Can you work these out from the model? Positions are in its coordinate system, mm. Face numbers are marked on the shaded views. A direction names the side the tool comes from. Give positions to 0.01 mm unless a question says otherwise; leave off trailing zeros. Write each loop counter-clockwise with the first axis right and the second up, starting at its lowest first coordinate (ties: lowest second). Pieces come first, ordered by that corner, then holes.
```python
from build123d import *

# Parameters (mm, degrees)
SKETCH1_W           = 54
SKETCH1_H           = 26.5
BOSS_EXTRUDE1_DEPTH = 9
SKETCH2_W           = 6
SKETCH2_H           = 15
BOSS_EXTRUDE2_DEPTH = 19
SKETCH4_R           = 2.06
CUT_EXTRUDE1_DEPTH  = 19
SKETCH5_R           = 2.06
BOSS_EXTRUDE3_DEPTH = 15
SKETCH8_W           = 54
SKETCH8_H           = 10
BOSS_EXTRUDE5_DEPTH = 9
SKETCH9_R           = 2.25
CUT_EXTRUDE3_DEPTH  = 15
FILLET1_R           = 2
FILLET2_R           = 1


with BuildPart() as part:
    # Sketch1 → Boss-Extrude1 (new body)
    with BuildSketch(Plane.XY):
        Rectangle(SKETCH1_W, SKETCH1_H)
    boss_extrude1 = extrude(amount=BOSS_EXTRUDE1_DEPTH)

    # Sketch2 → Boss-Extrude2 (add)
    with BuildSketch(Plane.XY.offset(9)):
        with Locations((24, 5.75)):
            Rectangle(SKETCH2_W, SKETCH2_H)
    boss_extrude2 = extrude(amount=BOSS_EXTRUDE2_DEPTH)

    # Sketch4 → Cut-Extrude1 (cut)
    with BuildSketch(Plane(origin=(0, 13.25, 0), x_dir=(1, 0, 0), z_dir=(0, 1, 0))):
        with Locations((23.9, -13.949454959)):
            Circle(SKETCH4_R)
        with Locations((23.9, -24.149454959)):
            Circle(SKETCH4_R)
    cut_extrude1 = extrude(amount=-CUT_EXTRUDE1_DEPTH, mode=Mode.SUBTRACT)

    # Sketch5 → Boss-Extrude3 (add)
    with BuildSketch(Plane(origin=(0, 13.25, 0), x_dir=(1, 0, 0), z_dir=(0, 1, 0))):
        with BuildLine():
            Line((21, -27.075954574), (21, -21.222955343))
            ThreePointArc((21, -21.222955343), (28.02, -24.149454959), (21, -27.075954574))
        make_face()
        with Locations((23.9, -24.149454959)):
            Circle(SKETCH5_R, mode=Mode.SUBTRACT)
        with BuildLine():
            Line((21, -16.875954574), (21, -11.022955343))
            ThreePointArc((21, -11.022955343), (28.02, -13.949454959), (21, -16.875954574))
        make_face()
        with Locations((23.9, -13.949454959)):
            Circle(SKETCH5_R, mode=Mode.SUBTRACT)
    boss_extrude3 = extrude(amount=-BOSS_EXTRUDE3_DEPTH)

    # Sketch8 → Boss-Extrude5 (add, through all)
    with BuildSketch(Plane.XY.offset(9)):
        with Locations((0, -18.25)):
            Rectangle(SKETCH8_W, SKETCH8_H)
    extrude(amount=-BOSS_EXTRUDE5_DEPTH)

    # Sketch9 → Cut-Extrude3 (cut)
    with BuildSketch(Plane.XY.offset(9)):
        with Locations((19, -18.25)):
            Circle(SKETCH9_R)
        with Locations((-12, -18.25)):
            Circle(SKETCH9_R)
    extrude(amount=-CUT_EXTRUDE3_DEPTH, mode=Mode.SUBTRACT)

    # Mirror1: Boss-Extrude1, Boss-Extrude2, Cut-Extrude1, Boss-Extrude3 across plane
    add(boss_extrude1.mirror(Plane.ZY))
    add(boss_extrude2.mirror(Plane.ZY))
    add(cut_extrude1.mirror(Plane.ZY), mode=Mode.SUBTRACT)
    add(boss_extrude3.mirror(Plane.ZY))

    # Fillet1
    fillet1_edges = [part.edges().sort_by_distance(p)[0] for p in [
        (-24, -1.75, 9),
        (24, -1.75, 9),
    ]]
    fillet(fillet1_edges, radius=FILLET1_R)

    # Fillet2
    fillet2_edges = [part.edges().sort_by_distance(p)[0] for p in [
        (-21, 5.75, 9),
        (21, 5.75, 9),
    ]]
    fillet(fillet2_edges, radius=FILLET2_R)


solid = part.part
```
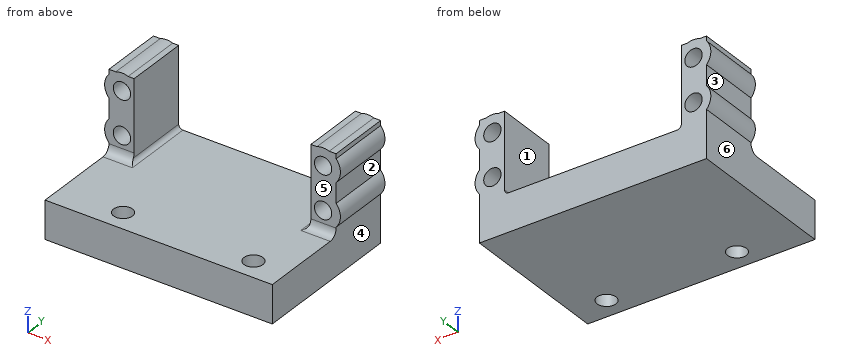
1) Please list where these lines run through material, in increasing order: L1, parallel to Z at x = -23.9, y = 6.75; L2, parallel to Z at x = 23, y = 8; L3, parallel to Y at x = -12, z = 3.75.
Values follow:
L1: z = 0 to 11.89, 16.01 to 22.09, 26.21 to 28.27
L2: z = 0 to 12.1, 15.8 to 22.3, 26 to 28.17
L3: y = -23.25 to -20.5, -16 to 13.25
2) Suppose I cut it at B-B on z = 19. Write out the boundary of the cut face in (x, y), plus the area to 3 significant figures.
Values follow:
outline: (-27, -1.75) - (-21, -1.75) - (-21, 13.25) - (-27, 13.25) - close; (21, -1.75) - (27, -1.75) - (27, 13.25) - (21, 13.25) - close
area: 180 mm2
3) If we mould it in two halves opening along X, with no side actions, what happens to the marked faces 1, 2 and 3? For each: +X half, -X half, draft (parallel to the pull), parting line (faces both ways), or undercut.
Values follow:
face 1: undercut
face 2: +X half
face 3: -X half
4) Suppose I cut it at C-C on y = -18.25. Write out the boundary of the cut face in (x, z), plus the area to 3 significant figures.
Values follow:
outline: (-27, 0) - (-14.25, 0) - (-14.25, 9) - (-27, 9) - close; (-9.75, 0) - (16.75, 0) - (16.75, 9) - (-9.75, 9) - close; (21.25, 0) - (27, 0) - (27, 9) - (21.25, 9) - close
area: 405 mm2
5) For the marked faces 4, 5 and 6, which set-ups out of +Z, -Z, +X, -X, +Y, -Y let a thin tool reach every point of the face, with its end or its side?
Values follow:
face 4: -Z, +X, +Y, -Y
face 5: +Z, +X, -X, -Y
face 6: -Z, -X, +Y, -Y
6) For pin 1 Ø3.5 at (x, z) = (23.5, 20) entering from -Y; pin 2 Ø2 at (x, y) = (12, -10) entering from +Z; pin 3 Ø6 at (x, y) = (1, -13.5) entering from -Z; pin 4 Ø5.5 at (y, z) = (-5, 8) entering from -X, each with a flat end and sliding along its axis, tell me the tip position at first contact or that it passes through.
Values follow:
pin 1: stops at y = -1.75
pin 2: stops at z = 9
pin 3: stops at z = 0
pin 4: stops at x = -27
7) Suppose I cut it at A-A on x = -23.9. Write out the boundary of the cut face in (y, z).
Values follow:
outline: (-23.25, 0) - (13.25, 0) - (13.25, 11.89) - (-1.75, 11.89) - (-1.75, 11) arc R2 cw to (-3.75, 9) - (-23.25, 9) - close; (-1.75, 16.01) - (13.25, 16.01) - (13.25, 22.09) - (-1.75, 22.09) - close; (-1.75, 26.21) - (13.25, 26.21) - (13.25, 28.27) - (-1.75, 28.27) - close
8) Suppose I cut it at D-D on x = -12. Write out the boundary of the cut face in (y, z), plus the area to 3 significant figures.
Values follow:
outline: (-23.25, 0) - (-20.5, 0) - (-20.5, 9) - (-23.25, 9) - close; (-16, 0) - (13.25, 0) - (13.25, 9) - (-16, 9) - close
area: 288 mm2
